```python
from build123d import *

# Parameters (mm, degrees)
F0_W     = 100
F0_H     = 100
F1_DEPTH = 100
F3_DEPTH = 100
F4_R     = 11.25
F5_DEPTH = 30
F6_W     = 10
F6_H     = 10
F7_DEPTH = 50


with BuildPart() as f1:
    # F0 (on Top) → F1 (new body)
    with BuildSketch(Plane.XY):
        with Locations((50, -50)):
            Rectangle(F0_W, F0_H)
    extrude(amount=F1_DEPTH)

    # F2 (on face) → F3 (cut)
    with BuildSketch(Plane.YZ.offset(100)):
        with BuildLine():
            Line((-88.576018, -5.630251), (-90, 0))
            Line((-90, 0), (-100, 10))
            Line((-100, 10), (-100, 40))
            ThreePointArc((-100, 40), (-97.071068, 47.071068), (-90, 50))
            Line((-90, 50), (-50, 50))
            Line((-50, 50), (-50, 85))
            Line((-50, 85), (-35, 100))
            Line((-35, 100), (-35, 130.032703))
            Line((-35, 130.032703), (-148.719932, 130.032703))
            Line((-148.719932, 130.032703), (-148.719932, -5.630251))
            Line((-148.719932, -5.630251), (-88.576018, -5.630251))
        make_face()
    extrude(amount=-F3_DEPTH, mode=Mode.SUBTRACT)

    # F4 (on face) → F5 (cut)
    with BuildSketch(Plane.YZ.offset(100)):
        with Locations((-25, 60)):
            Circle(F4_R)
        with Locations((-25, 30)):
            Circle(F4_R)
    extrude(amount=-F5_DEPTH, mode=Mode.SUBTRACT)

    # F6 (on face) → F7 (cut)
    with BuildSketch(Plane.XY.offset(50)):
        with Locations((25, -70)):
            Rectangle(F6_W, F6_H)
        with Locations((50, -70)):
            Rectangle(F6_W, F6_H)
        with Locations((75, -70)):
            Rectangle(F6_W, F6_H)
    extrude(amount=-F7_DEPTH, mode=Mode.SUBTRACT)


solid = f1.part
```
CAD build for the part. Positions are in the model's coordinates, mm. A direction names the side the tool comes from. Round coordinates to 2 decimals unless told otherwise and drop trailing zeros. Order: outer loops, then holes, each group sorted by start corner. A loop starts at its lowest first (then second) coordinate and runs counter-clockwise, first axis right, second up.
Q1. Two-plate mould, pull along Y, no slides. Class faces 1 (the cylindrical face through (50.7, -97.15, 46.99)), 2 (the flat face through (70, -70, 25)), 3 (the flat face through (0, -40, 38)): pulls with the +Y half, pulls with the -Y half, needs draft (parallel to the pull), parting line crosses it, or undercut.
Q2. Drop flat-ended pins along their axis: pin 1 (1 mm diameter, centred on x = 13.5, z = 49.5, fed in from -Y); pin 2 (12 mm diameter, centred on x = 68, y = -75, fed in from +Z); pin 3 (10 mm diameter, centred on y = -44.5, z = 69, fed in from -X); pin 4 (1.5 mm diameter, centred on x = 21, z = 83, fed in from -Y). Give the stop position or say it passes through.
Q3. Slice it at B-B (z = 7.5). Write the cut outline in (x, y), and give its area (3 significant figures).
Q4. Slice it at C-C (y = -68). Write the cut outline in (x, z), and give its area (3 significant figures).
Q5. Slice it at D-D (x = 39.5). Write the cut outline in (y, z), and give its area (3 significant figures).
Q6. Wall check: L1, parallel to Z at x = 93.25, y = -25; L2, parallel to Y at x = 78.5, z = 60.5; L3, parallel to Y at x = 75.5, z = 16. Give the ranges that are in metal, low to high.
Q7. Which spindle directions (+Z, -Z, +X, -X, +Y, -Y) get a long thin tool onto all of the face, cutting with end or side? Do faces 4 (the flat face through (51, -79, 50)), 5 (the flat face through (49, -17, 100)), 6 (the cylindrical face through (85.21, -18.952, 39.486)), 7 (the flat face through (30, -70, 25)). Say none if no direction does.
Q8. Slice it at A-A (x = 76.5). Write the cut outline in (y, z), and give its area (3 significant figures).
Results below:
1. face 1: pulls with the -Y half
1. face 2: undercut
1. face 3: needs draft
2. pin 1: stops at y = -94.36
2. pin 2: stops at z = 50
2. pin 3: stops at x = 0
2. pin 4: stops at y = -50
3. outline: (0, -97.5) - (100, -97.5) - (100, 0) - (0, 0) - close; hole (20, -75) - (30, -75) - (30, -65) - (20, -65) - close; hole (45, -75) - (55, -75) - (55, -65) - (45, -65) - close; hole (70, -75) - (80, -75) - (80, -65) - (70, -65) - close
3. area: 9,450 mm2
4. outline: (0, 0) - (20, 0) - (20, 50) - (0, 50) - close; (30, 0) - (45, 0) - (45, 50) - (30, 50) - close; (55, 0) - (70, 0) - (70, 50) - (55, 50) - close; (80, 0) - (100, 0) - (100, 50) - (80, 50) - close
4. area: 3,500 mm2
5. outline: (-100, 10) - (-90, 0) - (0, 0) - (0, 100) - (-35, 100) - (-50, 85) - (-50, 50) - (-90, 50) arc R10 ccw to (-100, 40) - close
5. area: 7,320 mm2
6. L1: z = 0 to 18.75, 41.25 to 48.75, 71.25 to 100
6. L2: y = -50 to -36.24, -13.76 to 0
6. L3: y = -100 to -75, -65 to 0
7. face 4: +Z, +X, -X, -Y
7. face 5: +Z, +X, -X, +Y, -Y
7. face 6: +X
7. face 7: +Z, -Z
8. outline: (-100, 10) - (-90, 0) - (-75, 0) - (-75, 50) - (-90, 50) arc R10 ccw to (-100, 40) - close; (-65, 0) - (0, 0) - (0, 100) - (-35, 100) - (-50, 85) - (-50, 50) - (-65, 50) - close; hole circle Ø22.5 at (-25, 30); hole circle Ø22.5 at (-25, 60)
8. area: 6,020 mm2
